For this review, take the finished solid that the model builds, in its own axes (mm). A direction names the side the tool comes from. Round coordinates to 2 decimals unless told otherwise and drop trailing zeros. Order: outer loops, then holes, each group sorted by start corner. A loop starts at its lowest first (then second) coordinate and runs counter-clockwise, first axis right, second up. Notation, with made-up numbers: (39, 62.5) -> (92, 62.5) arc R24 ccw to (92, 75.5) -> close; hole circle Ø4 at (3.5, -10.5). An arc over 180 degrees is marked (long way). Answer in a Markdown table with one row per item.
```python
from build123d import *

# Parameters (mm, degrees)
SKETCH_R     = 2
PAD_DEPTH    = 1
SKETCH001_W  = 14
SKETCH001_H  = 77
PAD001_DEPTH = 3
SKETCH002_W  = 12
SKETCH002_H  = 75
POCKET_DEPTH = 2
SKETCH003_W  = 5
SKETCH003_H  = 5
PAD002_DEPTH = 2


with BuildPart() as part:
    # Sketch → Pad (new body)
    with BuildSketch(Plane.XY):
        with BuildLine():
            Line((7, 38.5), (7, -38.5))
            Line((7, -38.5), (4, -38.5))
            Line((4, -38.5), (4, -41.5))
            ThreePointArc((-4, -41.5), (0, -45.5), (4, -41.5))
            Line((-4, -38.5), (-4, -41.5))
            Line((-7, -38.5), (-4, -38.5))
            Line((-7, 38.5), (-7, -38.5))
            Line((-7, 38.5), (-4, 38.5))
            Line((-4, 41.5), (-4, 38.5))
            ThreePointArc((4, 41.5), (0, 45.500017), (-4, 41.5))
            Line((4, 41.5), (4, 38.5))
            Line((4, 38.5), (7, 38.5))
        make_face()
        with Locations((0, -41.5)):
            Circle(SKETCH_R, mode=Mode.SUBTRACT)
        with Locations((0, 41.500017)):
            Circle(SKETCH_R, mode=Mode.SUBTRACT)
    extrude(amount=PAD_DEPTH)

    # Sketch001 → Pad001 (join)
    with BuildSketch(Plane.XY):
        Rectangle(SKETCH001_W, SKETCH001_H)
    extrude(amount=PAD001_DEPTH)

    # Sketch002 (on Face17 of Pad001) → Pocket (cut)
    with BuildSketch(Plane.XY.offset(3)):
        Rectangle(SKETCH002_W, SKETCH002_H)
    extrude(amount=-POCKET_DEPTH, mode=Mode.SUBTRACT)

    # Sketch003 → Pad002 (join)
    with BuildSketch(Plane.XY):
        with Locations((0, 28)):
            Rectangle(SKETCH003_W, SKETCH003_H)
        with Locations((0, 14)):
            Rectangle(SKETCH003_W, SKETCH003_H)
        Rectangle(SKETCH003_W, SKETCH003_H)
        with Locations((0, -14)):
            Rectangle(SKETCH003_W, SKETCH003_H)
        with Locations((0, -28)):
            Rectangle(SKETCH003_W, SKETCH003_H)
    extrude(amount=PAD002_DEPTH)


solid = part.part
```
Q1. Clearance check with flat-ended pins moving along their axes: pin 1 Ø1.6 at (x, z) = (-1.5, 2) entering from +Y; pin 2 Ø5.5 at (x, y) = (1.5, 42) entering from +Z; pin 3 Ø1.1 at (x, z) = (-0.5, 1.5) entering from -Y; pin 4 Ø8 at (x, y) = (-5, -29.5) entering from +Z. State where each tip first meets the part, or that it passes through.
Answer key:
| item | result |
|---|---|
| pin 1 | stops at y = 38.5 |
| pin 2 | stops at z = 1 |
| pin 3 | stops at y = -45.49 |
| pin 4 | stops at z = 3 |
Q2. Tool access review of faces 1 (the face through (7, 1, 1)), 2 (the face through (-6, -1, 2)): name each direction out of +Z, -Z, +X, -X, +Y, -Y from which nothing blocks a thin tool from reaching the whole face with its end or side.
Answer key:
| item | result |
|---|---|
| face 1 | +Z, -Z, +X, +Y, -Y |
| face 2 | +Z |
Q3. To check wall thickness, follow probe 1 along Y at (x, z) = (0, 0.8); probe 2 along X at (y, z) = (-10.5, 1.8); probe 3 along Y at (x, z) = (-3.5, 1.75). State the ranges of each line that lie inside material, in increasing order.
Answer key:
| item | result |
|---|---|
| probe 1 | y = -45.5 to -43.5, -39.5 to 39.5, 43.5 to 45.5 |
| probe 2 | x = -7 to -6, 6 to 7 |
| probe 3 | y = -38.5 to -37.5, 37.5 to 38.5 |
Q4. Take a section at A-A, the plane y = 28. Write out the cut boundary in (x, z).
Answer key:
| item | result |
|---|---|
| outline | (-7, 0) -> (7, 0) -> (7, 3) -> (6, 3) -> (6, 1) -> (2.5, 1) -> (2.5, 2) -> (-2.5, 2) -> (-2.5, 1) -> (-6, 1) -> (-6, 3) -> (-7, 3) -> close |
Q5. Take a section at B-B, the plane z = 2.5. Write out the cut boundary in (x, y), then the cut area to 3 significant figures.
Answer key:
| item | result |
|---|---|
| outline | (-7, -38.5) -> (7, -38.5) -> (7, 38.5) -> (-7, 38.5) -> close; hole (-6, -37.5) -> (6, -37.5) -> (6, 37.5) -> (-6, 37.5) -> close |
| area | 178 mm^2 |
Q6. Take a section at C-C, the plane x = 5.25. Write out the cut boundary in (y, z).
Answer key:
| item | result |
|---|---|
| outline | (-38.5, 0) -> (38.5, 0) -> (38.5, 3) -> (37.5, 3) -> (37.5, 1) -> (-37.5, 1) -> (-37.5, 3) -> (-38.5, 3) -> close |
Q7. The part is to be moulded in two halves that separate along X. For faces 3 (the face through (-7, 1, 1)), 4 (the face through (6, -1, 2)), 5 (the face through (0, -44, 1)), 6 (the face through (0, -37.5, 2)), say which applies: +X half, -X half, draft (parallel to the pull), parting line (faces both ways), or undercut.
Answer key:
| item | result |
|---|---|
| face 3 | -X half |
| face 4 | undercut |
| face 5 | draft |
| face 6 | undercut |
Q8. Take a section at D-D, the plane x = 0. Give the number of separate pieces and of enclosed holes in the cut face, then the cut area to 3 significant figures.
Answer key:
| item | result |
|---|---|
| separate pieces | 3 |
| enclosed holes | 0 |
| area | 112 mm^2 |
